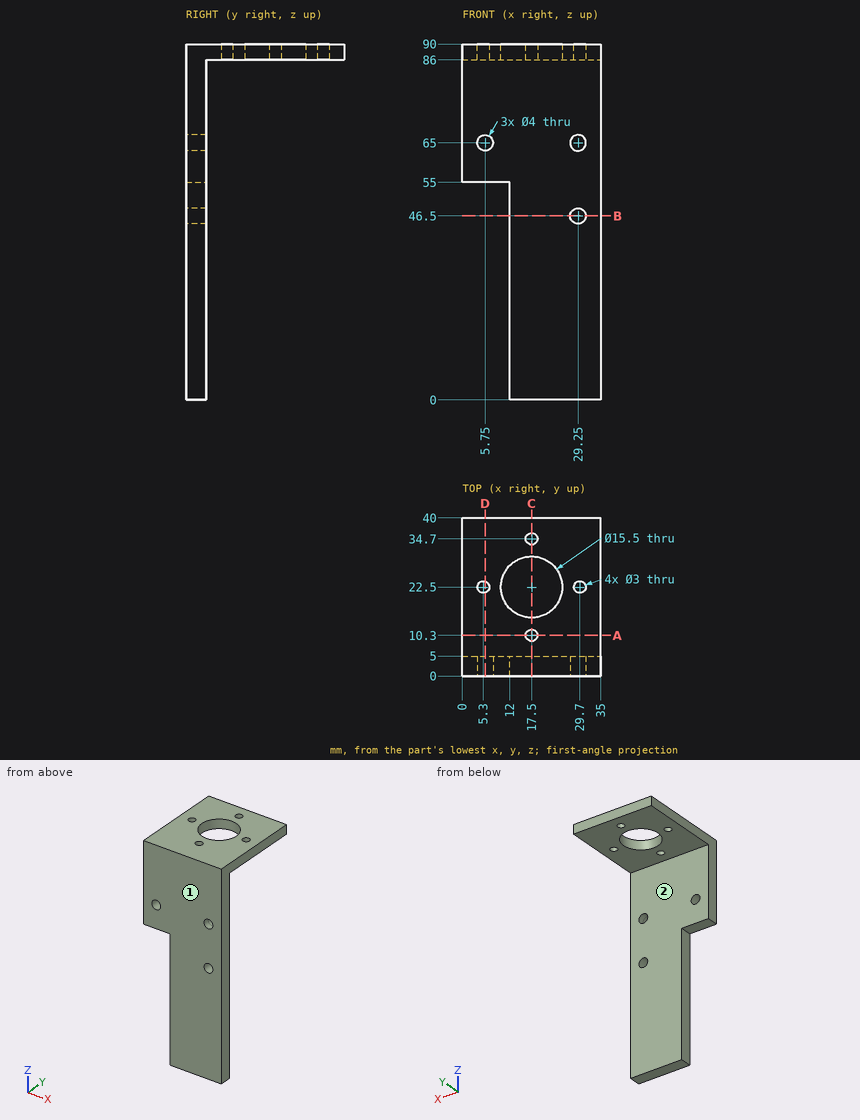
Could you check a few things on this drawing? It's one solid part, dimensions in mm from its lowest x, y, z. A direction names the side the tool comes from. Give positions to 0.01 mm unless a question says otherwise; leave off trailing zeros. Write each loop counter-clockwise with the first axis right and the second up, starting at its lowest first coordinate (ties: lowest second). Pieces come first, ordered by that corner, then holes. Notation, with made-up numbers: M 34,15 L 45,15 A6 cw 45,22 Z; hole C 48.25,86.5 d11. An arc over 180 degrees is marked long. Put each result on its own line as item: value. Start each with the question number.
Item 1: If we section it at C-C, the plane x = 17.5: Write out the boundary of the cut face in (y, z).
Item 2: If we section it at D-D, the plane x = 5.75: Write out the boundary of the cut face in (y, z), then the cut area to 3 significant figures.
Item 3: If we section it at A-A, the plane y = 10.3: Write out the boundary of the cut face in (x, z), then the cut area to 3 significant figures.
Item 4: On a 3-axis mill with a long thin cutter (end or side, diameter ignored), from which of +Z, -Z, +X, -X, +Y, -Y can I reach the whole of each face in a straight line? I mean the marked faces 1 and 2. Say none if no direction works.
Item 5: I need wall thicknesses on L1, parallel to Y at x = 17.5, z = 88; L2, parallel to X at y = 2, z = 65; L3, parallel to Z at x = 29, y = 1. Which ranges of each line are inside material? Lowest first, please. Write a range as from..to.
Item 6: Will these pins go through, and if not, where does the flat tip stop? pin 1 (2.5 mm diameter, centred on x = 29.25, z = 65, fed in from +Y); pin 2 (3.5 mm diameter, centred on x = 29.7, y = 22.5, fed in from -Z); pin 3 (8 mm diameter, centred on x = 23.5, z = 19, fed in from -Y); pin 4 (1.5 mm diameter, centred on x = 6.5, y = 3.5, fed in from -Z).
Item 7: If we section it at B-B, the plane z = 46.5: Write out the boundary of the cut face in (x, y), then the cut area to 3 significant figures.
Values:
1. outline: M 0,0 L 5,0 L 5,86 L 8.8,86 L 8.8,90 L 0,90 Z; M 11.8,86 L 14.75,86 L 14.75,90 L 11.8,90 Z; M 30.25,86 L 33.2,86 L 33.2,90 L 30.25,90 Z; M 36.2,86 L 40,86 L 40,90 L 36.2,90 Z
2. outline: M 0,55 L 5,55 L 5,63 L 0,63 Z; M 0,67 L 5,67 L 5,86 L 21.07,86 L 21.07,90 L 0,90 Z; M 23.93,86 L 40,86 L 40,90 L 23.93,90 Z
2. area: 284 mm²
3. outline: M 0,86 L 16,86 L 16,90 L 0,90 Z; M 19,86 L 35,86 L 35,90 L 19,90 Z
3. area: 128 mm²
4. face 1: +Z, -Z, +X, -X, -Y
4. face 2: -Z, +X, -X, +Y
5. L1: 0..8.8, 11.8..14.75, 30.25..33.2, 36.2..40
5. L2: 0..3.75, 7.75..27.25, 31.25..35
5. L3: 0..44.52, 48.48..63.02, 66.98..90
6. pin 1: through
6. pin 2: z = 86
6. pin 3: y = 0
6. pin 4: z = 55
7. outline: M 12,0 L 27.25,0 L 27.25,5 L 12,5 Z; M 31.25,0 L 35,0 L 35,5 L 31.25,5 Z
7. area: 95.0 mm²
